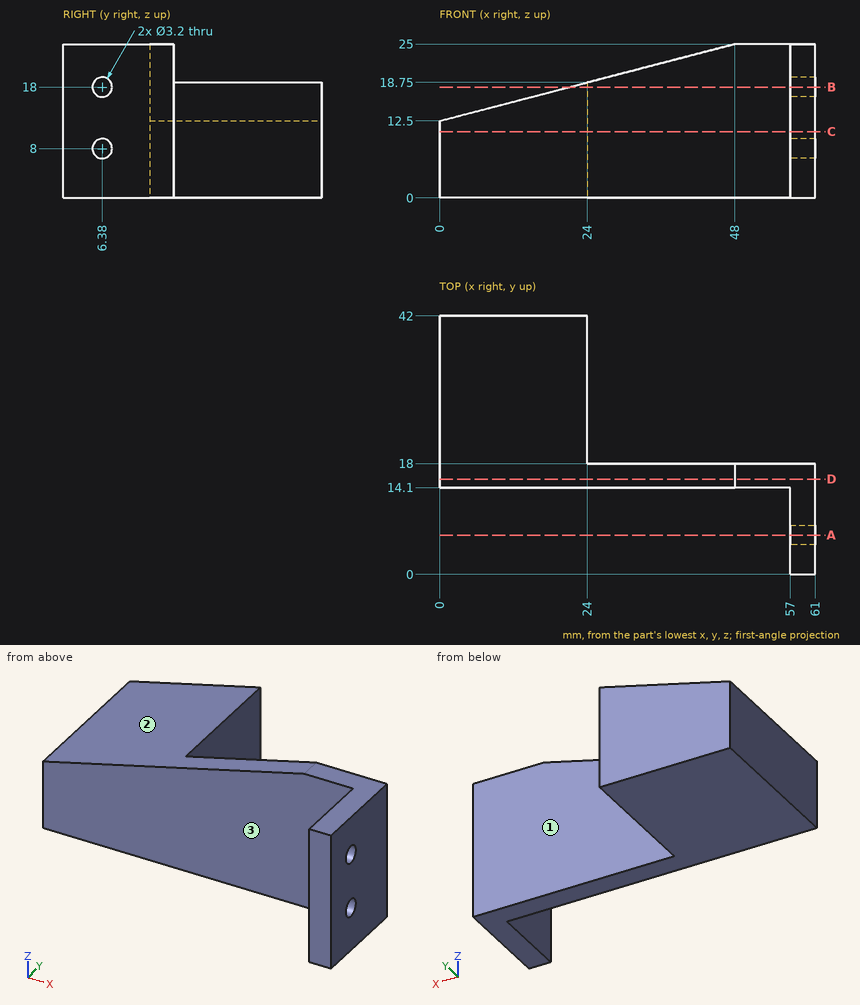
Here's the drawing with two shaded views (mm, measured from the low corner). I have some questions. A direction names the side the tool comes from. Round coordinates to 2 decimals unless told otherwise and drop trailing zeros. Order: outer loops, then holes, each group sorted by start corner. A loop starts at its lowest first (then second) coordinate and runs counter-clockwise, first axis right, second up. Notation, with made-up numbers: M 74.25,-26 L 111.25,-26 A18 cw 111.25,-21 Z; hole C -39,57.5 d9. An arc over 180 degrees is marked long. Use CSV: the item, a comma, the result in double quotes.
1) I'm going to push flat-ended pins straight in: P1, Ø1.9, axis at y = 6.38, z = 18, coming from the +X side; P2, Ø7.5, axis at x = 51.5, z = 13.5, coming from the +Y side; P3, Ø11.5, axis at y = 8, z = 6.5, coming from the -X side; P4, Ø9.5, axis at y = 24.5, z = 11, coming from the +X side. Where does each tip first touch, or does it pass through?
Taken from the geometry:
P1,"through"
P2,"y = 18"
P3,"x = 57"
P4,"x = 24"
2) I want a section at B-B (z = 18). List the corners of the cut face in (x, y) for me.
Taken from the geometry:
outline,"M 21.12,14.1 L 57,14.1 L 57,7.98 L 61,7.98 L 61,18 L 24,18 L 24,42 L 21.12,42 Z; M 57,0 L 61,0 L 61,4.78 L 57,4.78 Z"
3) On a 3-axis mill with a long thin cutter (end or side, diameter ignored), from which of +Z, -Z, +X, -X, +Y, -Y can I reach the whole of each face in a straight line? I mean the marked faces 1, 2 and 3. Say none if no direction works.
Taken from the geometry:
face 1,"+Z, -Z, +X, +Y"
face 2,"+Z, -X, +Y, -Y"
face 3,"+Z, -Z, -X, -Y"
4) I want a section at A-A (y = 6.38). List the corners of the cut face in (x, z) for me, then the cut area to 3 significant figures.
Taken from the geometry:
outline,"M 57,0 L 61,0 L 61,6.4 L 57,6.4 Z; M 57,9.6 L 61,9.6 L 61,16.4 L 57,16.4 Z; M 57,19.6 L 61,19.6 L 61,25 L 57,25 Z"
area,"74.4 mm^2"
5) I want a section at C-C (z = 10.75). List the corners of the cut face in (x, y) for me.
Taken from the geometry:
outline,"M 0,14.1 L 57,14.1 L 57,0 L 61,0 L 61,18 L 24,18 L 24,42 L 0,42 Z"
6) I want a section at D-D (y = 15.5). List the corners of the cut face in (x, z) for me, then the cut area to 4 significant figures.
Taken from the geometry:
outline,"M 0,0 L 61,0 L 61,25 L 48,25 L 0,12.5 Z"
area,"1,225 mm^2"
7) I need wall thicknesses on line 1 along Z through (x, y) = (58.2, 6.38); line 2 along Y through (x, z) = (18, 6.25); line 3 along X through (y, z) = (4, 23). Which ranges of each line are inside material? Lowest first, please. Write a range as [from, to].
Taken from the geometry:
line 1,"[0, 6.4], [9.6, 16.4], [19.6, 25]"
line 2,"[14.1, 42]"
line 3,"[57, 61]"
